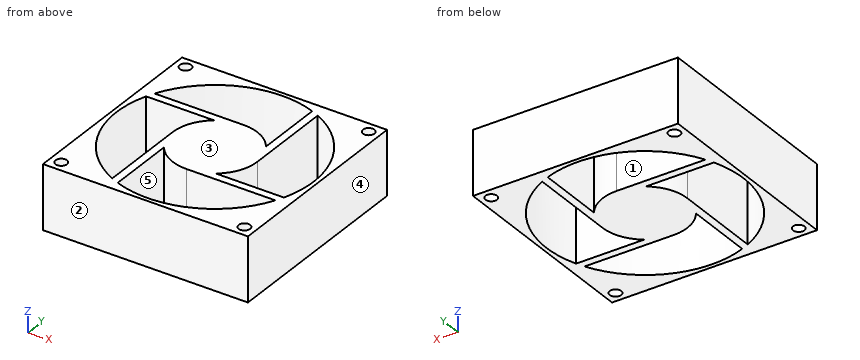
from build123d import *

# Parameters (mm, degrees)
F0_W     = 80
F0_H     = 80
F0_R     = 2.25
F0_R_2   = 38.5
F1_DEPTH = 25
F3_DEPTH = 25


with BuildPart() as f1:
    # F0 (on Top) → F1 (new body)
    with BuildSketch(Plane.XY):
        Rectangle(F0_W, F0_H)
        with Locations((-35.75, -35.75)):
            Circle(F0_R, mode=Mode.SUBTRACT)
        with Locations((35.75, -35.75)):
            Circle(F0_R, mode=Mode.SUBTRACT)
        with Locations((-35.75, 35.75)):
            Circle(F0_R, mode=Mode.SUBTRACT)
        Circle(F0_R_2, mode=Mode.SUBTRACT)
        with Locations((35.75, 35.75)):
            Circle(F0_R, mode=Mode.SUBTRACT)
    extrude(amount=F1_DEPTH)

    # F2 (on Top) → F3 (join)
    with BuildSketch(Plane.XY):
        with BuildLine():
            ThreePointArc((9.4868329805, -13.5), (14.6421095505, -7.6064859108), (16.5, 0))
            Line((16.5, 0), (13.5, 0))
            Line((13.5, 0), (13.5, 9.4868329805))
            ThreePointArc((13.5, 9.4868329805), (7.6064859108, 14.6421095505), (0, 16.5))
            Line((0, 16.5), (0, 13.5))
            Line((0, 13.5), (-9.4868329805, 13.5))
            ThreePointArc((-9.4868329805, 13.5), (-14.6421095505, 7.6064859108), (-16.5, 0))
            Line((-16.5, 0), (-13.5, 0))
            Line((-13.5, 0), (-13.5, -9.4868329805))
            ThreePointArc((-13.5, -9.4868329805), (-7.6064859108, -14.6421095505), (0, -16.5))
            Line((0, -16.5), (0, -13.5))
            Line((0, -13.5), (9.4868329805, -13.5))
        make_face()
        with BuildLine():
            ThreePointArc((13.5, 9.4868329805), (15.7321327226, 4.9749371855), (16.5, 0))
            Line((16.5, 0), (16.5, 34.7850542619))
            ThreePointArc((16.5, 34.7850542619), (15.0134445147, 35.452030743), (13.5, 36.0555127546))
            Line((13.5, 36.0555127546), (13.5, 9.4868329805))
        make_face()
        with BuildLine():
            Line((13.5, 0), (16.5, 0))
            ThreePointArc((16.5, 0), (15.7321327226, 4.9749371855), (13.5, 9.4868329805))
            Line((13.5, 9.4868329805), (13.5, 0))
        make_face()
        with BuildLine():
            Line((0, 13.5), (0, 16.5))
            ThreePointArc((0, 16.5), (-4.9749371855, 15.7321327226), (-9.4868329805, 13.5))
            Line((-9.4868329805, 13.5), (0, 13.5))
        make_face()
        with BuildLine():
            ThreePointArc((-9.4868329805, 13.5), (-4.9749371855, 15.7321327226), (0, 16.5))
            Line((0, 16.5), (-34.7850542619, 16.5))
            ThreePointArc((-34.7850542619, 16.5), (-35.452030743, 15.0134445147), (-36.0555127546, 13.5))
            Line((-36.0555127546, 13.5), (-9.4868329805, 13.5))
        make_face()
        with BuildLine():
            ThreePointArc((-16.5, 0), (-15.7321327226, -4.9749371855), (-13.5, -9.4868329805))
            Line((-13.5, -9.4868329805), (-13.5, 0))
            Line((-13.5, 0), (-16.5, 0))
        make_face()
        with BuildLine():
            Line((-13.5, -36.0555127546), (-13.5, -9.4868329805))
            ThreePointArc((-13.5, -9.4868329805), (-15.7321327226, -4.9749371855), (-16.5, 0))
            Line((-16.5, 0), (-16.5, -34.7850542619))
            ThreePointArc((-16.5, -34.7850542619), (-15.0134445147, -35.452030743), (-13.5, -36.0555127546))
        make_face()
        with BuildLine():
            ThreePointArc((0, -16.5), (4.9749371855, -15.7321327226), (9.4868329805, -13.5))
            Line((9.4868329805, -13.5), (0, -13.5))
            Line((0, -13.5), (0, -16.5))
        make_face()
        with BuildLine():
            Line((36.0555127546, -13.5), (9.4868329805, -13.5))
            ThreePointArc((9.4868329805, -13.5), (4.9749371855, -15.7321327226), (0, -16.5))
            Line((0, -16.5), (34.7850542619, -16.5))
            ThreePointArc((34.7850542619, -16.5), (35.452030743, -15.0134445147), (36.0555127546, -13.5))
        make_face()
    extrude(amount=F3_DEPTH)


solid = f1.part
Read the model definition and answer for the solid it produces. Units are mm, in the model's axes. Face numbers are marked on the shaded views. A direction names the side the tool comes from. Give positions to 0.01 mm unless a question says otherwise; leave off trailing zeros. Loops run counter-clockwise (first coordinate to the right, second up) from the corner with the lowest first, then second, coordinate; pieces in that order, holes last. Notation, with made-up numbers: (47, -24) - (78, -24) arc R33 ccw to (78, 13) - close; hole circle Ø8 at (66, -24.75). An arc over 180 degrees is marked (long way). Answer as CSV lines item,"result". Start each with the question number.
1) Straight lines are drawn through the part: L1, parallel to Y at x = 24.5, z = 7.75; L2, parallel to X at y = 21.5, z = 2.5; L3, parallel to Y at x = -5, z = 12.75. For each, find the intervals that lie inside material, in ascending order. Write a range as from..to.
2) Find section B-B (x = -28). Write down the section's boundary in (y, z).
3) Determine the mould class of the marked faces 3, 4 and 5 for opening direction X: released by +X, released by -X, zero draft, split by the parting line, or undercut.
4) Find section C-C (y = 21). Write down the section's boundary in (x, z).
5) Find section A-A (z = 20.25). State how many separate pieces and enclosed holes the cut face has, then the cut area to 3 significant figures.
6) Which of the six approach directions +Z, -Z, +X, -X, +Y, -Y give full straight-line access (tool end or side, diameter ignored) to the marked faces 1 and 2?
Findings below:
1,L1,"-40..-29.7, -16.5..-13.5, 29.7..40"
1,L2,"-40..-31.94, 13.5..16.5, 31.94..40"
1,L3,"-40..-38.17, -15.72..16.5, 38.17..40"
2,outline,"(-40, 0) - (-26.42, 0) - (-26.42, 25) - (-40, 25) - close; (13.5, 0) - (16.5, 0) - (16.5, 25) - (13.5, 25) - close; (26.42, 0) - (40, 0) - (40, 25) - (26.42, 25) - close"
3,face 3,"zero draft"
3,face 4,"released by +X"
3,face 5,"undercut"
4,outline,"(-40, 0) - (-32.27, 0) - (-32.27, 25) - (-40, 25) - close; (13.5, 0) - (16.5, 0) - (16.5, 25) - (13.5, 25) - close; (32.27, 0) - (40, 0) - (40, 25) - (32.27, 25) - close"
5,separate pieces,"1"
5,enclosed holes,"8"
5,area,"2,880 mm^2"
6,face 1,"+Z, -Z"
6,face 2,"+Z, -Z, +X, -X, -Y"
